Source: CAD feature listing. Evaluate the final solid. Frame: model axes, mm. Face numbers are marked on the shaded views. A direction names the side the tool comes from. Round coordinates to 2 decimals unless told otherwise and drop trailing zeros. Write each loop counter-clockwise with the first axis right and the second up, starting at its lowest first coordinate (ties: lowest second). Pieces come first, ordered by that corner, then holes. Notation, with made-up numbers: M 53,61 L 61,61 A12 cw 61,84 Z; hole C 5,-16.5 d4. An arc over 180 degrees is marked long. Answer in a Markdown table with one row per item.
from build123d import *

# Parameters (mm, degrees)
BOSS_EXTRUDE1_DEPTH      = 125
BOSS_EXTRUDE1_DEPTH_BACK = 125
SKETCH1_W                = 50
SKETCH1_H                = 30
CUT_EXTRUDE1_DEPTH       = 254.031618578
CUT_EXTRUDE2_DEPTH       = 254.031618578
CUT_EXTRUDE3_DEPTH       = 254.031618578
SKETCH6_R                = 2.05
CUT_EXTRUDE4_DEPTH       = 6
CUT_EXTRUDE5_DEPTH       = 253.477691783
BOSS_EXTRUDE2_DEPTH      = 250
BOSS_EXTRUDE3_DEPTH      = 250
CUT_EXTRUDE6_DEPTH       = 253.477691783
SKETCH11_W               = 16
SKETCH11_H               = 10
CUT_EXTRUDE7_DEPTH       = 4
SKETCH12_W               = 16
SKETCH12_H               = 18
CUT_EXTRUDE11_DEPTH      = 4
BOSS_EXTRUDE4_DEPTH      = 250
CUT_EXTRUDE12_DEPTH      = 4
SKETCH15_W               = 30
SKETCH15_H               = 2
BOSS_EXTRUDE5_DEPTH      = 250
FILLET1_R                = 4
FILLET2_R                = 3
SKETCH16_R               = 2.05
CUT_EXTRUDE13_DEPTH      = 6
SKETCH17_R               = 2.05
CUT_EXTRUDE14_DEPTH      = 6
SKETCH18_R               = 2.05
CUT_EXTRUDE15_DEPTH      = 6


with BuildPart() as part:
    # Sketch1 → Boss-Extrude1 (new, two sides: drawn at the far end of the back side and taken through both)
    with BuildSketch(Plane(origin=(0, 0, 0), x_dir=(0, 0, -1), z_dir=(1, 0, 0)).offset(-BOSS_EXTRUDE1_DEPTH_BACK)):
        with Locations((0, 15)):
            Rectangle(SKETCH1_W, SKETCH1_H)
    extrude(amount=BOSS_EXTRUDE1_DEPTH + BOSS_EXTRUDE1_DEPTH_BACK)

    # Sketch2 → Cut-Extrude1 (cut, through all)
    with BuildSketch(Plane(origin=(125, 0, 0), x_dir=(0, 0, -1), z_dir=(1, 0, 0))):
        Polygon((-10, 0), (-25, 15), (-25, 0), align=None)
        Polygon((25, 15), (10, 0), (25, 0), align=None)
    extrude(amount=-CUT_EXTRUDE1_DEPTH, mode=Mode.SUBTRACT)

    # Sketch4 → Cut-Extrude2 (cut, through all)
    with BuildSketch(Plane(origin=(125, 0, 0), x_dir=(0, 0, -1), z_dir=(1, 0, 0))):
        Polygon((-22.171572875, 12.171572875), (-19.343145751, 15), (-25, 20.656854249), (-25, 15), align=None)
        Polygon((22.171572875, 12.171572875), (19.343145751, 15), (25, 20.656854249), (25, 15), align=None)
    extrude(amount=-CUT_EXTRUDE2_DEPTH, mode=Mode.SUBTRACT)

    # Sketch5 → Cut-Extrude3 (cut, through all)
    with BuildSketch(Plane(origin=(125, 0, 0), x_dir=(0, 0, -1), z_dir=(1, 0, 0))):
        Polygon((-25, 20.656854249), (-20.757359313, 24.899494937), (-15, 19.142135624), (15, 19.142135624), (20.757359313, 24.899494937), (25, 20.656854249), (25, 30), (-25, 30), align=None)
    extrude(amount=-CUT_EXTRUDE3_DEPTH, mode=Mode.SUBTRACT)

    # Sketch6 → Cut-Extrude4 (cut)
    with BuildSketch(Plane(origin=(0, 19.142135624, 0), x_dir=(1, 0, 0), z_dir=(0, 1, 0))):
        with Locations(Location((-10, 0, 0), (0, 0, 270))):
            Circle(SKETCH6_R)
        with Locations(Location((10, 0, 0), (0, 0, 270))):
            Circle(SKETCH6_R)
        with Locations(Location((30, 0, 0), (0, 0, 270))):
            Circle(SKETCH6_R)
        with Locations(Location((50, 0, 0), (0, 0, 270))):
            Circle(SKETCH6_R)
        with Locations(Location((70, 0, 0), (0, 0, 270))):
            Circle(SKETCH6_R)
        with Locations(Location((90, 0, 0), (0, 0, 270))):
            Circle(SKETCH6_R)
        with Locations(Location((-30, 0, 0), (0, 0, 270))):
            Circle(SKETCH6_R)
        with Locations(Location((-50, 0, 0), (0, 0, 270))):
            Circle(SKETCH6_R)
        with Locations(Location((-70, 0, 0), (0, 0, 270))):
            Circle(SKETCH6_R)
        with Locations(Location((-90, 0, 0), (0, 0, 270))):
            Circle(SKETCH6_R)
    extrude(amount=-CUT_EXTRUDE4_DEPTH, mode=Mode.SUBTRACT)

    # Sketch7 → Cut-Extrude5 (cut, through all)
    with BuildSketch(Plane.ZY.offset(125)):
        Polygon((-8.343145751, 4), (-2, 4), (-2, 10.647041832), (-6.495093791, 15.142135624), (-10.495093791, 15.142135624), (-14.990187583, 10.647041832), align=None)
        Polygon((8.343145751, 4), (14.990187583, 10.647041832), (10.495093791, 15.142135624), (6.495093791, 15.142135624), (2, 10.647041832), (2, 4), align=None)
    extrude(amount=-CUT_EXTRUDE5_DEPTH, mode=Mode.SUBTRACT)

    # Sketch8 → Boss-Extrude2 (add, through all)
    with BuildSketch(Plane.ZY.offset(125)):
        Polygon((-12, 13.637229415), (-12, 7.656854249), (-14.990187583, 10.647041832), align=None)
        Polygon((12, 13.637229415), (12, 7.656854249), (14.990187583, 10.647041832), align=None)
    extrude(amount=-BOSS_EXTRUDE2_DEPTH)

    # Sketch9 → Boss-Extrude3 (add, through all)
    with BuildSketch(Plane(origin=(125, 0, 0), x_dir=(0, 0, -1), z_dir=(1, 0, 0))):
        Polygon((-16.085786438, 6.085786438), (16.085786438, 6.085786438), (10, 0), (-10, 0), align=None)
    extrude(amount=-BOSS_EXTRUDE3_DEPTH)

    # Sketch10 → Cut-Extrude6 (cut, through all)
    with BuildSketch(Plane(origin=(125, 0, 0), x_dir=(0, 0, -1), z_dir=(1, 0, 0))):
        Polygon((-12.085786438, 2.085786438), (12.085786438, 2.085786438), (10, 0), (-10, 0), align=None)
    extrude(amount=-CUT_EXTRUDE6_DEPTH, mode=Mode.SUBTRACT)

    # Sketch11 → Cut-Extrude7 (cut)
    with BuildSketch(Plane(origin=(0, -5, 5), x_dir=(1, 0, 0), z_dir=(0, -0.7071067811865477, 0.7071067811865475))):
        with Locations((117, 19.284271247)):
            Rectangle(SKETCH11_W, SKETCH11_H)
        with Locations((-117, 19.284271247)):
            Rectangle(SKETCH11_W, SKETCH11_H)
    extrude(amount=-CUT_EXTRUDE7_DEPTH, mode=Mode.SUBTRACT)

    # Sketch12 → Cut-Extrude11 (cut)
    with BuildSketch(Plane(origin=(0, -5, -5), x_dir=(-1, 0, 0), z_dir=(0, -0.7071067811865477, -0.7071067811865475))):
        with Locations((-117, 23.284271247)):
            Rectangle(SKETCH12_W, SKETCH12_H)
        with Locations((117, 23.284271247)):
            Rectangle(SKETCH12_W, SKETCH12_H)
    extrude(amount=-CUT_EXTRUDE11_DEPTH, mode=Mode.SUBTRACT)

    # Sketch13 → Boss-Extrude4 (add, through all)
    with BuildSketch(Plane(origin=(125, 0, 0), x_dir=(0, 0, -1), z_dir=(1, 0, 0))):
        Polygon((7.600505063, 6.085786438), (13.514718626, 12), (14.928932188, 10.585786438), (10.428932188, 6.085786438), align=None)
        Polygon((-7.600505063, 6.085786438), (-13.514718626, 12), (-14.928932188, 10.585786438), (-10.428932188, 6.085786438), align=None)
    extrude(amount=-BOSS_EXTRUDE4_DEPTH)

    # Sketch14 → Cut-Extrude12 (cut)
    with BuildSketch(Plane(origin=(0, 19.142135624, 0), x_dir=(1, 0, 0), z_dir=(0, 1, 0))):
        Polygon((125, 11), (109, 0), (125, -11), align=None)
        Polygon((-125, 11), (-109, 0), (-125, -11), align=None)
    extrude(amount=-CUT_EXTRUDE12_DEPTH, mode=Mode.SUBTRACT)

    # Sketch15 → Boss-Extrude5 (add, through all)
    with BuildSketch(Plane.ZY.offset(125)):
        with Locations((0, 14.142135624)):
            Rectangle(SKETCH15_W, SKETCH15_H)
    extrude(amount=-BOSS_EXTRUDE5_DEPTH)

    # Fillet1
    fillet1_edges = [part.edges().sort_by_distance(p)[0] for p in [
        (109, 17.142135624, 0),
        (-109, 17.142135624, 0),
    ]]
    fillet(fillet1_edges, radius=FILLET1_R)

    # Fillet2
    fillet2_edges = [part.edges().sort_by_distance(p)[0] for p in [
        (109, 6.514718626, 13.686291501),
        (-109, 6.514718626, 13.686291501),
        (109, 6.514718626, -13.686291501),
        (-109, 6.514718626, -13.686291501),
    ]]
    fillet(fillet2_edges, radius=FILLET2_R)

    # Sketch16 → Cut-Extrude13 (cut)
    with BuildSketch(Plane(origin=(0, 15.142135624, 0), x_dir=(1, 0, 0), z_dir=(0, 1, 0))):
        with Locations(Location((119, 0, 0), (0, 0, 270))):
            Circle(SKETCH16_R)
        with Locations(Location((-119, 0, 0), (0, 0, 270))):
            Circle(SKETCH16_R)
    extrude(amount=-CUT_EXTRUDE13_DEPTH, mode=Mode.SUBTRACT)

    # Sketch17 → Cut-Extrude14 (cut)
    with BuildSketch(Plane(origin=(0, -2.171572875, -2.171572875), x_dir=(-1, 0, 0), z_dir=(0, -0.7071067811865469, -0.7071067811865481))):
        with Locations(Location((-115, 19.284271247, 0), (0, 0, 90))):
            Circle(SKETCH17_R)
        with Locations(Location((115, 19.284271247, 0), (0, 0, 90))):
            Circle(SKETCH17_R)
    extrude(amount=-CUT_EXTRUDE14_DEPTH, mode=Mode.SUBTRACT)

    # Sketch18 → Cut-Extrude15 (cut)
    with BuildSketch(Plane(origin=(0, -2.171572875, 2.171572875), x_dir=(1, 0, 0), z_dir=(0, -0.7071067811865477, 0.7071067811865475))):
        with Locations(Location((-115, 19.284271247, 0), (0, 0, 270))):
            Circle(SKETCH18_R)
        with Locations(Location((115, 19.284271247, 0), (0, 0, 270))):
            Circle(SKETCH18_R)
    extrude(amount=-CUT_EXTRUDE15_DEPTH, mode=Mode.SUBTRACT)


solid = part.part
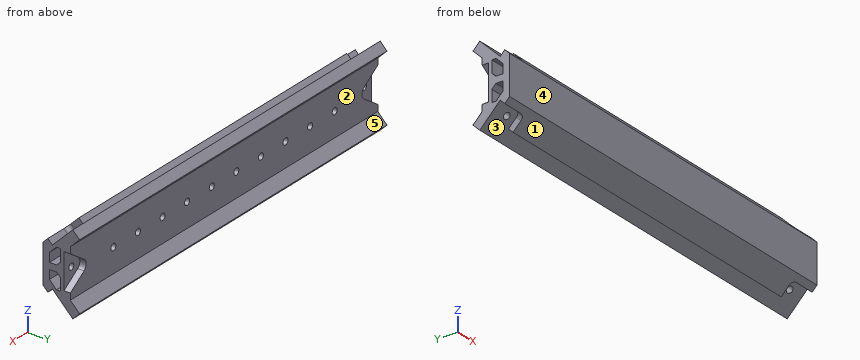
Q1. Pull-direction query (Y, two-part tool) for the marked faces 1, 2 and 3; classes: pulls with the +Y half, pulls with the -Y half, needs draft (parallel to the pull), parting line crosses it, or undercut.
Solutions:
| item | result |
|---|---|
| face 1 | pulls with the -Y half |
| face 2 | pulls with the +Y half |
| face 3 | undercut |
Q2. Material intervals for probe 1 along Y at (x, z) = (-89.5, -6.5); probe 2 along Z at (x, y) = (-26, 9.75); probe 3 along Y at (x, z) = (-98.5, 9.5), sorted ascending.
Solutions:
| item | result |
|---|---|
| probe 1 | y = 2.09 to 6.09, 13.14 to 19.14 |
| probe 2 | z = -19.75 to -11.26, -2 to 2, 11.26 to 19.75 |
| probe 3 | y = 2.09 to 7.99, 13.14 to 19.14 |
Q3. Access query for the marked faces 4 and 5. Directions: +Z, -Z, +X, -X, +Y, -Y. A direction counts if a zero-diameter tool reaches every point of the face in a straight line with its end or side. Return the directions, or none.
Solutions:
| item | result |
|---|---|
| face 4 | +Z, -Z, +X, -X, -Y |
| face 5 | +X, -X, +Y |
Q4. Section B-B (x = -70). Return loops of the section in (y, z), and give its area (3 significant figures).
Solutions:
| item | result |
|---|---|
| outline | M 2.09,-12.09 L 12.17,-22.17 L 15,-19.34 L 20.66,-25 L 24.9,-20.76 L 19.14,-15 L 19.14,-2.05 L 15.14,-2.05 L 15.14,2.05 L 19.14,2.05 L 19.14,15 L 24.9,20.76 L 20.66,25 L 15,19.34 L 12.17,22.17 L 2.09,12.09 Z; hole M 6.09,-7.6 L 10.49,-12 L 13.14,-12 L 13.14,-4.5 L 10.65,-2 L 6.09,-2 Z; hole M 6.09,2 L 10.65,2 L 13.14,4.5 L 13.14,12 L 10.49,12 L 6.09,7.6 Z |
| area | 570 mm2 |
Q5. Section A-A (x = 74.5). Return loops of the section in (y, z).
Solutions:
| item | result |
|---|---|
| outline | M 2.09,-12.09 L 12.17,-22.17 L 15,-19.34 L 20.66,-25 L 24.9,-20.76 L 19.14,-15 L 19.14,15 L 24.9,20.76 L 20.66,25 L 15,19.34 L 12.17,22.17 L 2.09,12.09 Z; hole M 6.09,-7.6 L 10.49,-12 L 13.14,-12 L 13.14,-4.5 L 10.65,-2 L 6.09,-2 Z; hole M 6.09,2 L 10.65,2 L 13.14,4.5 L 13.14,12 L 10.49,12 L 6.09,7.6 Z |
Q6. Contact query for flat-ended pins moving along their axis: pin 1 Ø6 at (x, z) = (-55, 4) entering from +Y; pin 2 Ø10 at (x, y) = (63.5, 22.5) entering from -Z; pin 3 Ø2 at (x, z) = (118, 0) entering from +Y; pin 4 Ø2 at (y, z) = (21.5, 11) entering from +X. Output: stop coordinate, or through.
Solutions:
| item | result |
|---|---|
| pin 1 | stops at y = 19.14 |
| pin 2 | stops at z = -25 |
| pin 3 | stops at y = 9.14 |
| pin 4 | passes through |
